```python
from build123d import *

# Parameters (mm, degrees)
BOSS_EXTRUDE1_DEPTH                          = 10
FILLET1_R                                    = 3
CBORE_FOR_M3_HEX_HEAD_CAP_SCREW1_D           = 3.4
CBORE_FOR_M3_HEX_HEAD_CAP_SCREW1_CBORE_D     = 7
CBORE_FOR_M3_HEX_HEAD_CAP_SCREW1_CBORE_DEPTH = 8


with BuildPart() as part:
    # Sketch1 → Boss-Extrude1 (new body)
    with BuildSketch(Plane(origin=(0, 0, 0), x_dir=(0, 0, -1), z_dir=(1, 0, 0))):
        Polygon((215, 5), (-205, 5), (-215, -5), (205, -5), align=None)
        Polygon((-165.5, -3), (-205.5, -3), (-199.5, 3), (-159.5, 3), align=None, mode=Mode.SUBTRACT)
        Polygon((-160.25, -3), (-154.25, 3), (-114.25, 3), (-120.25, -3), align=None, mode=Mode.SUBTRACT)
        Polygon((-115, -3), (-109, 3), (-69, 3), (-75, -3), align=None, mode=Mode.SUBTRACT)
        Polygon((-69.75, -3), (-63.75, 3), (-23.75, 3), (-29.75, -3), align=None, mode=Mode.SUBTRACT)
        Polygon((-24.5, -3), (-18.5, 3), (21.5, 3), (15.5, -3), align=None, mode=Mode.SUBTRACT)
        Polygon((20.75, -3), (26.75, 3), (66.75, 3), (60.75, -3), align=None, mode=Mode.SUBTRACT)
        Polygon((66, -3), (72, 3), (112, 3), (106, -3), align=None, mode=Mode.SUBTRACT)
        Polygon((111.25, -3), (117.25, 3), (157.25, 3), (151.25, -3), align=None, mode=Mode.SUBTRACT)
        Polygon((156.5, -3), (162.5, 3), (202.5, 3), (196.5, -3), align=None, mode=Mode.SUBTRACT)
    extrude(amount=BOSS_EXTRUDE1_DEPTH)

    # Fillet1
    fillet1_edges = [part.edges().sort_by_distance(p)[0] for p in [
        (5, -5, 215),
        (5, 5, 205),
        (5, -5, -205),
        (5, 5, -215),
        (5, -3, -156.5),
        (5, -3, -151.25),
        (5, 3, -162.5),
        (5, 3, -157.25),
        (5, -3, -106),
        (5, -3, -111.25),
        (5, 3, -112),
        (5, 3, -117.25),
        (5, -3, -66),
        (5, -3, -60.75),
        (5, 3, -72),
        (5, 3, -66.75),
        (5, -3, -15.5),
        (5, -3, -20.75),
        (5, 3, -21.5),
        (5, 3, -26.75),
        (5, -3, 24.5),
        (5, -3, 29.75),
        (5, 3, 18.5),
        (5, 3, 23.75),
        (5, -3, 75),
        (5, -3, 69.75),
        (5, 3, 69),
        (5, 3, 63.75),
        (5, -3, 115),
        (5, -3, 120.25),
        (5, 3, 109),
        (5, 3, 114.25),
        (5, -3, 160.25),
        (5, 3, 159.5),
        (5, 3, 154.25),
        (5, -3, 205.5),
        (5, 3, 199.5),
        (5, -3, -196.5),
        (5, 3, -202.5),
        (5, -3, 165.5),
    ]]
    fillet(fillet1_edges, radius=FILLET1_R - 0.0001)  # a hair under: the kernel refuses the full size

    # CBORE for M3 Hex Head Cap Screw1 (through all)
    with Locations(Plane(origin=(0, 5, 0), x_dir=(1, 0, 0), z_dir=(0, 1, 0))):
        with Locations((5, -210), (5, 0), (5, -107.5), (5, 107.5), (5, 210)):
            CounterBoreHole(CBORE_FOR_M3_HEX_HEAD_CAP_SCREW1_D / 2, CBORE_FOR_M3_HEX_HEAD_CAP_SCREW1_CBORE_D / 2, CBORE_FOR_M3_HEX_HEAD_CAP_SCREW1_CBORE_DEPTH)


solid = part.part
```
Check sheet for the modelled part. Datum: model origin and axes. Units: mm. A direction names the side the tool comes from. Round coordinates to 2 decimals unless told otherwise and drop trailing zeros. Order: outer loops, then holes, each group sorted by start corner. A loop starts at its lowest first (then second) coordinate and runs counter-clockwise, first axis right, second up. Notation, with made-up numbers: M -18,-18.5 L 41,-18.5 A26 ccw 41,13.5 Z; hole C -16,74.5 d3. An arc over 180 degrees is marked long. Answer in a Markdown table with one row per item.
(1) Draft check along Y on faces 1 (the flat face through (5, -3, 93)), 2 (the flat face through (5, 5, -5)), 3 (the flat face through (0, 3.4, 3)). Enter one of: +Y half, -Y half, draft (parallel to the pull), parting line (faces both ways), or undercut.
Findings:
| item | result |
|---|---|
| face 1 | undercut |
| face 2 | +Y half |
| face 3 | draft |
(2) Set-up check for faces 4 (the flat face through (5, -3, 137)), 5 (the cylindrical face through (8.34, 4.01, -1.05)): record each of +Z, -Z, +X, -X, +Y, -Y from which the full face is reachable in a straight line by a thin tool's end or side.
Findings:
| item | result |
|---|---|
| face 4 | +X, -X |
| face 5 | +Y |
(3) Gauge pin test, flat ends, axial feed: pin 1 (2.5 mm diameter, centred on x = 5, z = 210, fed in from +Y); pin 2 (1 mm diameter, centred on x = 8.5, y = 2.5, fed in from -Z); pin 3 (1.5 mm diameter, centred on x = 4.5, y = -1.5, fed in from -Z); pin 4 (4 mm diameter, centred on x = 5, z = 210, fed in from -Y). Record the tip position at first contact, or that the pin passes through.
Findings:
| item | result |
|---|---|
| pin 1 | passes through |
| pin 2 | stops at z = -210.76 |
| pin 3 | stops at z = -206.73 |
| pin 4 | stops at y = -4.99 |
(4) Section check A-A on z = -100.5. Record the boundary of the cut face in (x, y), plus the area to 3 significant figures.
Findings:
| item | result |
|---|---|
| outline | M 0,-5 L 10,-5 L 10,-3 L 0,-3 Z; M 0,3 L 10,3 L 10,5 L 0,5 Z |
| area | 40.0 mm^2 |
(5) Material ranges on line 1 along Z through (x, y) = (5, -4.1); line 2 along Y through (x, z) = (4, -10.5); line 3 along Z through (x, y) = (5, 3.4), recorded low to high. Write a range as from..to.
Findings:
| item | result |
|---|---|
| line 1 | z = -205.9..-109.2, -105.8..-1.7, 1.7..105.8, 109.2..208.3 |
| line 2 | y = -5..-3, 3..5 |
| line 3 | z = -206.5..-111, -104..-3.5, 3.5..104, 111..206.5 |
